Work out the finished part from the listing and answer in its coordinate system (mm). A direction names the side the tool comes from. Round coordinates to 2 decimals unless told otherwise and drop trailing zeros. Loops run counter-clockwise (first coordinate to the right, second up) from the corner with the lowest first, then second, coordinate; pieces in that order, holes last. Notation, with made-up numbers: (-20.5, 9) - (31.5, 9) arc R25 cw to (31.5, 35) - close; hole circle Ø3 at (89, -19.5). An arc over 180 degrees is marked (long way). Answer as CSV lines item,"result". Start each with the question number.
Q1. Section C-C on y = -4 is taken. Write down the section's boundary in (x, z).
Q2. For faces 1 (the face through (0, 0, -7.01)), 2 (the face through (0.31, 2.33, -0.75)), 3 (the face through (3, 3, 18.466)), 4 (the face through (0, 0, 19.304)), determine the directions among +Z, -Z, +X, -X, +Y, -Y from which every point of the face is accessible in a straight line to the end or side of a thin tool.
Q3. Each of these flat-tipped pins is pushed along its axis until it touches: pin 1 Ø4 at (x, y) = (-5, -1.5) entering from -Z; pin 2 Ø1 at (y, z) = (-4.5, 3) entering from +X; pin 3 Ø1.5 at (x, y) = (1, 0.5) entering from +Z; pin 4 Ø1 at (x, z) = (-5, 16) entering from -Y. Where does it stop, or does it pass through?
Q4. Straight lines are drawn through the part: L1, parallel to Z at x = 3.5, y = 4.25; L2, parallel to Z at x = 0.25, y = 0.75; L3, parallel to X at y = -0.5, z = 19. For each, find the intervals that lie inside material, in ascending order. Write a range as [from, to].
Q5. Section A-A on x = 0 is taken. Write down the section's boundary in (y, z).
Q6. Section D-D on x = 3.25 is taken. Write down the section's boundary in (y, z).
Q7. The mould has two halves that part along Y. Classify faces 5 (the face through (0, 0.343, -4)), 6 (the face through (1, 1, -1.524)), 7 (the face through (-4.16, -0.41, 19.36)): +Y half, -Y half, draft (parallel to the pull), parting line (faces both ways), or undercut.
Q8. Section B-B on z = 16 is taken. Write down the section's boundary in (x, y).
```python
from build123d import *

# Parameters (mm, degrees)
EXTRUDE1_DEPTH     = 18.5928
SKETCH2_R          = 2.3495
EXTRUDE2_DEPTH     = 1.524
SKETCH3_R          = 0.74803
EXTRUDE3_DEPTH     = 5.4864
SKETCH4_R          = 2.5019
EXTRUDE4_DEPTH     = 0.7112
SKETCH6_R          = 0.806604734
SKETCH6_R_2        = 0.8001
CUT_EXTRUDE1_DEPTH = 2
CUT_EXTRUDE2_DEPTH = 0.7112
CUT_EXTRUDE3_DEPTH = 0.7112
EXTRUDE5_DEPTH     = 2.8702
FILLET1_R          = 0.254
SKETCH11_R         = 0.3556
CUT_EXTRUDE4_DEPTH = 0.381
SKETCH12_R         = 0.3556
CUT_EXTRUDE5_DEPTH = 0.381
SKETCH13_R         = 0.764641256
EXTRUDE6_DEPTH     = 0.127
SKETCH14_R         = 0.976393175
EXTRUDE7_DEPTH     = 0.127
EXTRUDE8_DEPTH     = 5.207


with BuildPart() as part:
    # Sketch1 → Extrude1 (new body)
    with BuildSketch(Plane.XY):
        with BuildLine():
            Line((-4.907461425, 5.9944), (4.907461425, 5.9944))
            ThreePointArc((4.907461425, 5.9944), (7.747, 0), (4.907461425, -5.9944))
            Line((4.907461425, -5.9944), (-4.907461425, -5.9944))
            ThreePointArc((-4.907461425, -5.9944), (-7.747, 0), (-4.907461425, 5.9944))
        make_face()
    extrude(amount=EXTRUDE1_DEPTH)

    # Sketch2 → Extrude2 (add)
    with BuildSketch(Plane(origin=(0, 0, 0), x_dir=(-1, 0, 0), z_dir=(0, 0, -1))):
        Circle(SKETCH2_R)
    extrude(amount=EXTRUDE2_DEPTH)

    # Sketch3 → Extrude3 (add)
    with BuildSketch(Plane(origin=(0, 0, -1.524), x_dir=(-1, 0, 0), z_dir=(0, 0, -1))):
        Circle(SKETCH3_R)
    extrude(amount=EXTRUDE3_DEPTH)

    # Sketch4 → Extrude4 (add)
    with BuildSketch(Plane.XY.offset(18.5928)):
        Circle(SKETCH4_R)
    extrude(amount=EXTRUDE4_DEPTH)

    # Sketch6 → Cut-Extrude1 (cut)
    with BuildSketch(Plane(origin=(0, 0, 0), x_dir=(-1, 0, 0), z_dir=(0, 0, -1))):
        with Locations((4.333417915, 2.5019)):
            Circle(SKETCH6_R)
        with Locations((-4.333417915, -2.5019)):
            Circle(SKETCH6_R_2)
    extrude(amount=-CUT_EXTRUDE1_DEPTH, mode=Mode.SUBTRACT)

    # Sketch8 → Cut-Extrude2 (cut)
    with BuildSketch(Plane.XY.offset(18.5928)):
        with BuildLine():
            Line((2.303011093, 0.97757021), (7.222442902, 3.065745123))
            Line((7.222442902, 3.065745123), (8.200013112, 0.76273403))
            Line((8.200013112, 0.76273403), (0.97757021, -2.303011093))
            ThreePointArc((0.97757021, -2.303011093), (2.319721286, -0.937228236), (2.303011093, 0.97757021))
        make_face()
    extrude(amount=-CUT_EXTRUDE2_DEPTH, mode=Mode.SUBTRACT)

    # Sketch9 → Cut-Extrude3 (cut)
    with BuildSketch(Plane.XY.offset(18.5928)):
        with BuildLine():
            Line((-2.303011093, -0.97757021), (-8.41785865, -3.573169003))
            Line((-8.41785865, -3.573169003), (-9.39542886, -1.27015791))
            Line((-9.39542886, -1.27015791), (-0.97757021, 2.303011093))
            ThreePointArc((-0.97757021, 2.303011093), (-2.319721286, 0.937228236), (-2.303011093, -0.97757021))
        make_face()
    extrude(amount=-CUT_EXTRUDE3_DEPTH, mode=Mode.SUBTRACT)

    # Sketch10 → Extrude5 (add)
    with BuildSketch(Plane.XY.offset(17.8816)):
        Polygon((-4.735400216, 0.169832597), (-4.149850547, -1.209635977), (-3.869280668, -1.090541129), (-4.454830337, 0.288927445), align=None)
        Polygon((3.869280668, 1.090541129), (4.149850547, 1.209635977), (4.735400216, -0.169832597), (4.454830337, -0.288927445), align=None)
    extrude(amount=EXTRUDE5_DEPTH)

    # Fillet1
    fillet1_edges = [part.edges().sort_by_distance(p)[0] for p in [
        (-4.595115277, 0.229380021, 20.7518),
        (-4.009565608, -1.150088553, 20.7518),
        (4.595115277, -0.229380021, 20.7518),
        (4.009565608, 1.150088553, 20.7518),
    ]]
    fillet(fillet1_edges, radius=FILLET1_R)

    # Sketch11 → Cut-Extrude4 (cut)
    with BuildSketch(Plane(origin=(-3.951359134, -1.677252442, 0), x_dir=(0, 0, 1), z_dir=(-0.920504853, -0.390731128, 0))):
        with Locations((20.001394918, 1.27)):
            Circle(SKETCH11_R)
    extrude(amount=-CUT_EXTRUDE4_DEPTH, mode=Mode.SUBTRACT)

    # Sketch12 → Cut-Extrude5 (cut)
    with BuildSketch(Plane(origin=(3.951359134, 1.677252442, 0), x_dir=(0, 0, -1), z_dir=(0.920504853, 0.390731128, 0))):
        with Locations((-19.9898, -1.2446)):
            Circle(SKETCH12_R)
    extrude(amount=-CUT_EXTRUDE5_DEPTH, mode=Mode.SUBTRACT)

    # Sketch13 → Extrude6 (add)
    with BuildSketch(Plane.XY.offset(17.8816)):
        with Locations((4.302340442, 0.460354266)):
            Circle(SKETCH13_R)
        with Locations((-4.302340442, -0.460354266)):
            Circle(SKETCH13_R)
    extrude(amount=EXTRUDE6_DEPTH)

    # Sketch14 → Extrude7 (cut)
    with BuildSketch(Plane.XY.offset(18.5928)):
        with Locations((3.109494983, 2.955380071)):
            Circle(SKETCH14_R)
    extrude(amount=-EXTRUDE7_DEPTH, mode=Mode.SUBTRACT)

    # Sketch15 → Extrude8 (cut)
    with BuildSketch(Plane(origin=(0, 0, -7.0104), x_dir=(-1, 0, 0), z_dir=(0, 0, -1))):
        with BuildLine():
            Line((-0.664807093, 0.3429), (0.664807093, 0.3429))
            ThreePointArc((0.664807093, 0.3429), (0, 0.74803), (-0.664807093, 0.3429))
        make_face()
    extrude(amount=-EXTRUDE8_DEPTH, mode=Mode.SUBTRACT)


solid = part.part
```
Findings:
1,outline,"(-6.63, 0) - (6.63, 0) - (6.63, 18.59) - (-6.63, 18.59) - close"
2,face 1,"-Z, +X, -X, +Y, -Y"
2,face 2,"-Z"
2,face 3,"+Z"
2,face 4,"+Z, +Y, -Y"
3,pin 1,"stops at z = 0"
3,pin 2,"stops at x = 6.63"
3,pin 3,"stops at z = 19.3"
3,pin 4,"stops at y = -5.99"
4,L1,"z = [0, 18.59]"
4,L2,"z = [-1.52, 19.3]"
4,L3,"x = [-4.45, -4.12], [-2.45, 2.45]"
5,outline,"(-5.99, 0) - (-2.35, 0) - (-2.35, -1.52) - (-0.75, -1.52) - (-0.75, -7.01) - (0.34, -7.01) - (0.34, -1.8) - (0.75, -1.8) - (0.75, -1.52) - (2.35, -1.52) - (2.35, 0) - (5.99, 0) - (5.99, 18.59) - (2.5, 18.59) - (2.5, 19.3) - (-2.5, 19.3) - (-2.5, 18.59) - (-5.99, 18.59) - close"
6,outline,"(-5.99, 0) - (5.99, 0) - (5.99, 18.59) - (3.92, 18.59) - (3.92, 18.47) - (1.99, 18.47) - (1.99, 18.59) - (1.38, 18.59) - (1.38, 17.88) - (-1.34, 17.88) - (-1.34, 18.59) - (-5.99, 18.59) - close"
7,face 5,"+Y half"
7,face 6,"draft"
7,face 7,"undercut"
8,outline,"(-4.91, -5.99) - (4.91, -5.99) arc R7.75 ccw to (4.91, 5.99) - (-4.91, 5.99) arc R7.75 ccw to start"
